Read the model definition and answer for the solid it produces. Units are mm, in the model's axes. A direction names the side the tool comes from. Coordinates: 2 decimals unless noted, no trailing zeros. Loops run counter-clockwise (first coordinate to the right, second up) from the corner with the lowest first, then second, coordinate; pieces in that order, holes last. Notation, with made-up numbers: (73, -31) -> (102, -31) arc R14 ccw to (102, -15) -> close; hole circle Ø11 at (9.25, -22.75). An arc over 180 degrees is marked (long way). Answer in a Markdown table with one row per item.
```python
from build123d import *

# Parameters (mm, degrees)
SKETCH2_W                = 290
SKETCH2_H                = 30
SKETCH2_W_2              = 280
SKETCH2_H_2              = 25
BOSS_EXTRUDE1_DEPTH      = 23.28
SKETCH3_W                = 290
SKETCH3_H                = 30
BOSS_EXTRUDE2_DEPTH      = 3
SKETCH4_W                = 23.28
SKETCH4_H                = 25
CUT_EXTRUDE1_DEPTH       = 1
CUT_EXTRUDE1_DEPTH_BACK  = 291
BOSS_EXTRUDE3_DEPTH      = 2
BOSS_EXTRUDE3_DEPTH_BACK = 3
SKETCH6_R                = 10
CUT_EXTRUDE2_DEPTH       = 2
SKETCH7_R                = 1.275
CUT_EXTRUDE3_DEPTH       = 10
SKETCH8_W                = 290
SKETCH8_H                = 2.5
CUT_EXTRUDE4_DEPTH       = 12
BOSS_EXTRUDE4_DEPTH      = 15


with BuildPart() as part:
    # Sketch2 → Boss-Extrude1 (new body)
    with BuildSketch(Plane.XY.offset(1.715456747)):
        Rectangle(SKETCH2_W, SKETCH2_H)
        Rectangle(SKETCH2_W_2, SKETCH2_H_2, mode=Mode.SUBTRACT)
    extrude(amount=BOSS_EXTRUDE1_DEPTH)

    # Sketch3 → Boss-Extrude2 (add)
    with BuildSketch(Plane.XY.offset(24.995456747)):
        Rectangle(SKETCH3_W, SKETCH3_H)
    extrude(amount=BOSS_EXTRUDE2_DEPTH)

    # Sketch4 → Cut-Extrude1 (cut, two sides)
    with BuildSketch(Plane(origin=(145, 0, 0), x_dir=(0, 0, -1), z_dir=(1, 0, 0))) as cut_extrude1_sk:
        with Locations((-13.355456747, 0)):
            Rectangle(SKETCH4_W, SKETCH4_H)
    extrude(amount=CUT_EXTRUDE1_DEPTH, mode=Mode.SUBTRACT)
    extrude(cut_extrude1_sk.sketch, amount=-CUT_EXTRUDE1_DEPTH_BACK, mode=Mode.SUBTRACT)

    # Sketch5 → Boss-Extrude3 (add, two sides)
    with BuildSketch(Plane(origin=(-0.5, 0, 0), x_dir=(0, 0, -1), z_dir=(1, 0, 0))) as boss_extrude3_sk:
        with BuildLine():
            Line((-27.995456747, 0), (-27.995456747, 15))
            Line((-27.995456747, 15), (-72.715456747, 15))
            Line((-72.715456747, 15), (-80.215456747, 0))
            Line((-80.215456747, 0), (-80.215456747, -21.531619709))
            ThreePointArc((-80.215456747, -21.531619709), (-72.715456747, -45.15), (-65.215456747, -21.531619709))
            Line((-65.215456747, -21.531619709), (-65.215456747, 0))
            Line((-65.215456747, 0), (-27.995456747, 0))
        make_face()
    extrude(amount=BOSS_EXTRUDE3_DEPTH)
    extrude(boss_extrude3_sk.sketch, amount=-BOSS_EXTRUDE3_DEPTH_BACK)

    # Sketch6 → Cut-Extrude2 (cut)
    with BuildSketch(Plane(origin=(-3.5, 0, 0), x_dir=(0, 0, -1), z_dir=(1, 0, 0))):
        with Locations((-72.715456747, -32.15)):
            Circle(SKETCH6_R)
    extrude(amount=CUT_EXTRUDE2_DEPTH, mode=Mode.SUBTRACT)

    # Sketch7 → Cut-Extrude3 (cut)
    with BuildSketch(Plane.ZY.offset(3.5)):
        with Locations((72.715456747, -25.15)):
            Circle(SKETCH7_R)
        with Locations((79.715456747, -32.15)):
            Circle(SKETCH7_R)
        with Locations((72.715456747, -39.15)):
            Circle(SKETCH7_R)
        with Locations((65.715456747, -32.15)):
            Circle(SKETCH7_R)
    extrude(amount=-CUT_EXTRUDE3_DEPTH, mode=Mode.SUBTRACT)

    # Sketch8 → Cut-Extrude4 (cut)
    with BuildSketch(Plane(origin=(0, 0, 1.715456747), x_dir=(-1, 0, 0), z_dir=(0, 0, -1))):
        with Locations((0, -13.75)):
            Rectangle(SKETCH8_W, SKETCH8_H)
    extrude(amount=-CUT_EXTRUDE4_DEPTH, mode=Mode.SUBTRACT)

    # Sketch9 → Boss-Extrude4 (add)
    with BuildSketch(Plane(origin=(0, 15, 0), x_dir=(1, 0, 0), z_dir=(0, 1, 0))):
        Polygon((-3.5, -58.92224084), (-63.5, -27.995456747), (-41.673741056, -27.995456747), (-3.5, -47.671974209), align=None)
        Polygon((61.5, -27.995456747), (39.673741056, -27.995456747), (1.5, -47.671974209), (1.5, -58.92224084), align=None)
    extrude(amount=-BOSS_EXTRUDE4_DEPTH)


solid = part.part
```
1. A cutting plane is placed at B-B on x = 11. Give the vertices of the cut face in (y, z).
A:
| item | result |
|---|---|
| outline | (-15, 13.72) -> (-12.5, 13.72) -> (-12.5, 25) -> (12.5, 25) -> (12.5, 1.72) -> (15, 1.72) -> (15, 28) -> (-15, 28) -> close; (0, 42.78) -> (15, 42.78) -> (15, 54.03) -> (0, 54.03) -> close |
2. A tool of negligible diameter and unlimited length cuts with its end or side. For faces 1 (the flat face through (2, -12.5, 19)), 2 (the flat face through (1.5, -15, 73)), 3 (the flat face through (-1, -11, 65.215)), 4 (the flat face through (-3.5, -15, 70)), 5 (the flat face through (20.85, 7.6, 37.7)), from which of +Z, -Z, +X, -X, +Y, -Y can it reach the whole face along a straight path? Write none if from no direction.
A:
| item | result |
|---|---|
| face 1 | -Z, +X, -X |
| face 2 | +Z, +X, +Y, -Y |
| face 3 | +X, -X |
| face 4 | +Z, -X, +Y, -Y |
| face 5 | +Y, -Y |
3. A cutting plane is placed at A-A on z = 38. Give the vertices of the cut face in (x, y).
A:
| item | result |
|---|---|
| outline | (-44.09, 0) -> (-22.26, 0) -> (-22.26, 15) -> (-44.09, 15) -> close; (-3.5, 0) -> (1.5, 0) -> (1.5, 15) -> (-3.5, 15) -> close; (20.26, 0) -> (42.09, 0) -> (42.09, 15) -> (20.26, 15) -> close |
4. Given pin 1 Ø3 at (y, z) = (1.5, 74) entering from -X; pin 2 Ø12.5 at (x, y) = (-28.5, -6) entering from -Z; pin 3 Ø3 at (y, z) = (-39.15, 72.72) entering from +X, each flat-ended and moving along its own axis, determine where each tip first touches the part or whether it passes through.
A:
| item | result |
|---|---|
| pin 1 | stops at x = -3.5 |
| pin 2 | stops at z = 25 |
| pin 3 | stops at x = 1.5 |
5. Find the intervals of material crossed by probe 1 along Z at (x, y) = (-2, -32); probe 2 along Z at (x, y) = (0, -32); probe 3 along X at (y, z) = (-14, 68), in increasing order.
A:
| item | result |
|---|---|
| probe 1 | z = 59.72 to 62.72, 82.71 to 85.71 |
| probe 2 | z = 59.72 to 64.45, 66.98 to 78.45, 80.98 to 85.71 |
| probe 3 | x = -3.5 to 1.5 |
6. The mould has two halves that part along X. Classify faces 6 (the flat face through (-1.5, -32, 73)), 7 (the flat face through (-3.5, 8, 38)), 8 (the flat face through (2, 15, 13)): pulls with the +X half, pulls with the -X half, needs draft (parallel to the pull), parting line crosses it, or undercut.
A:
| item | result |
|---|---|
| face 6 | pulls with the -X half |
| face 7 | undercut |
| face 8 | needs draft |
7. A cutting plane is placed at C-C on y = 10. Give the vertices of the cut face in (x, z), and give its area (3 significant figures).
A:
| item | result |
|---|---|
| outline | (-145, 25) -> (145, 25) -> (145, 28) -> (61.5, 28) -> (1.5, 58.92) -> (1.5, 75.22) -> (-3.5, 75.22) -> (-3.5, 58.92) -> (-63.5, 28) -> (-145, 28) -> close; hole (-41.67, 28) -> (-3.5, 28) -> (-3.5, 47.67) -> close; hole (1.5, 28) -> (39.67, 28) -> (1.5, 47.67) -> close |
| area | 2,210 mm2 |
8. A cutting plane is placed at D-D on x = -103.5. Give the vertices of the cut face in (y, z).
A:
| item | result |
|---|---|
| outline | (-15, 13.72) -> (-12.5, 13.72) -> (-12.5, 25) -> (12.5, 25) -> (12.5, 1.72) -> (15, 1.72) -> (15, 28) -> (-15, 28) -> close |
